```python
from build123d import *

# Parameters (mm, degrees)
SKETCH1_W                = 36
SKETCH1_H                = 110
BOSS_EXTRUDE1_DEPTH      = 1
F_4_0_4_DIAMETER_HOLE2_D = 4
F_4_0_4_DIAMETER_HOLE3_D = 4
F_4_0_4_DIAMETER_HOLE1_D = 4
BOSS_EXTRUDE2_DEPTH      = 1
FILLET1_R                = 4
CUT_EXTRUDE1_DEPTH       = 112.807870922
FILLET2_R                = 4


with BuildPart() as part:
    # Sketch1 → Boss-Extrude1 (new body)
    with BuildSketch(Plane(origin=(0, 0, 0), x_dir=(0, 0, -1), z_dir=(1, 0, 0))):
        with Locations((0, -55)):
            Rectangle(SKETCH1_W, SKETCH1_H)
    extrude(amount=BOSS_EXTRUDE1_DEPTH)

    # Ø4.0 (4) Diameter Hole2 (through all)
    with Locations(Plane.ZY):
        with Locations((-10, -8), (10, -8)):
            Hole(F_4_0_4_DIAMETER_HOLE2_D / 2)

    # Ø4.0 (4) Diameter Hole3 (through all)
    with Locations(Plane.ZY):
        with Locations((-13, -17), (13, -17)):
            Hole(F_4_0_4_DIAMETER_HOLE3_D / 2)

    # Ø4.0 (4) Diameter Hole1 (through all)
    with Locations(Plane(origin=(1, 0, 0), x_dir=(0, 0, -1), z_dir=(1, 0, 0))):
        with Locations((6, -94), (-6, -94)):
            Hole(F_4_0_4_DIAMETER_HOLE1_D / 2)

    # Sketch9 → Boss-Extrude2 (add)
    with BuildSketch(Plane.ZY):
        Polygon((18, -23.35), (20, -25.35), (20, -110), (18, -110), align=None)
        Polygon((-18, -23.35), (-20, -25.35), (-20, -110), (-18, -110), align=None)
    extrude(amount=-BOSS_EXTRUDE2_DEPTH)

    # Fillet1
    fillet1_edges = [part.edges().sort_by_distance(p)[0] for p in [
        (0.5, 0, 18),
        (0.5, 0, -18),
    ]]
    fillet(fillet1_edges, radius=FILLET1_R)

    # Sketch10 → Cut-Extrude1 (cut, through all)
    with BuildSketch(Plane.ZY):
        with BuildLine():
            Line((12, -86.75), (-12, -86.75))
            ThreePointArc((-12, -86.75), (-12.25, -86.5), (-12, -86.25))
            Line((-12, -86.25), (12, -86.25))
            ThreePointArc((12, -86.25), (12.25, -86.5), (12, -86.75))
        make_face()
        with BuildLine():
            Line((12, -26.75), (-12, -26.75))
            ThreePointArc((-12, -26.75), (-12.25, -26.5), (-12, -26.25))
            Line((-12, -26.25), (12, -26.25))
            ThreePointArc((12, -26.25), (12.25, -26.5), (12, -26.75))
        make_face()
    extrude(amount=-CUT_EXTRUDE1_DEPTH, mode=Mode.SUBTRACT)

    # Fillet2
    fillet2_edges = [part.edges().sort_by_distance(p)[0] for p in [
        (0.5, -25.35, 20),
        (0.5, -110, 20),
        (0.5, -110, -20),
        (0.5, -25.35, -20),
    ]]
    fillet(fillet2_edges, radius=FILLET2_R)


solid = part.part
```
For this review, take the finished solid that the model builds, in its own axes (mm). Round coordinates to 2 decimals unless told otherwise and drop trailing zeros. Write each loop counter-clockwise with the first axis right and the second up, starting at its lowest first coordinate (ties: lowest second). Pieces come first, ordered by that corner, then holes. Notation, with made-up numbers: (87, 4) -> (139, 4) arc R19 ccw to (139, 26) -> close; hole circle Ø3 at (39.25, 63.25). An arc over 180 degrees is marked (long way). One line per question, with ' | ' between items. Start each with the question number.
1) Wall thickness on line 1 along Y through (x, z) = (0.35, -6); line 2 along Y through (x, z) = (0.8, 1); line 3 along Y through (x, z) = (0.65, -10): over which ranges is each line inside the solid? List them lowest first.
2) Add section B-B (z = -6). Write out the cut boundary in (x, y), and give its area (3 significant figures).
3) Add section C-C (x = 0.7). Count the separate pieces of the cut face and the enclosed holes in it, and give its area (3 significant figures).
4) Mouldability with a two-part tool opening along Z and no side actions: class faces 1 (the flat face through (0, -54, 0)), 2 (the cylindrical face through (0.507, -1.141, -16.797)), 3 (the cylindrical face through (0.493, -92.017, -6.26)) as +Z half, -Z half, draft (parallel to the pull), parting line (faces both ways), or undercut.
5) Add section A-A (y = -17). Write out the cut boundary in (x, z).
6) For pin 1 Ø3.5 at (y, z) = (-8, -10) entering from +X; pin 2 Ø0.5 at (x, y) = (0.5, -14) entering from -Z, all flat-tipped, find the tip position at first contact; note any pin that passes through.
Reported:
1) line 1: y = -110 to -96, -92 to -86.75, -86.25 to -26.75, -26.25 to 0 | line 2: y = -110 to -86.75, -86.25 to -26.75, -26.25 to 0 | line 3: y = -110 to -86.75, -86.25 to -26.75, -26.25 to -10, -6 to 0
2) outline: (0, -110) -> (1, -110) -> (1, -96) -> (0, -96) -> close; (0, -92) -> (1, -92) -> (1, -86.75) -> (0, -86.75) -> close; (0, -86.25) -> (1, -86.25) -> (1, -26.75) -> (0, -26.75) -> close; (0, -26.25) -> (1, -26.25) -> (1, 0) -> (0, 0) -> close | area: 105 mm²
3) separate pieces: 1 | enclosed holes: 8 | area: 4,190 mm²
4) face 1: draft | face 2: -Z half | face 3: undercut
5) outline: (0, -18) -> (1, -18) -> (1, -15) -> (0, -15) -> close; (0, -11) -> (1, -11) -> (1, 11) -> (0, 11) -> close; (0, 15) -> (1, 15) -> (1, 18) -> (0, 18) -> close
6) pin 1: passes through | pin 2: stops at z = -18
